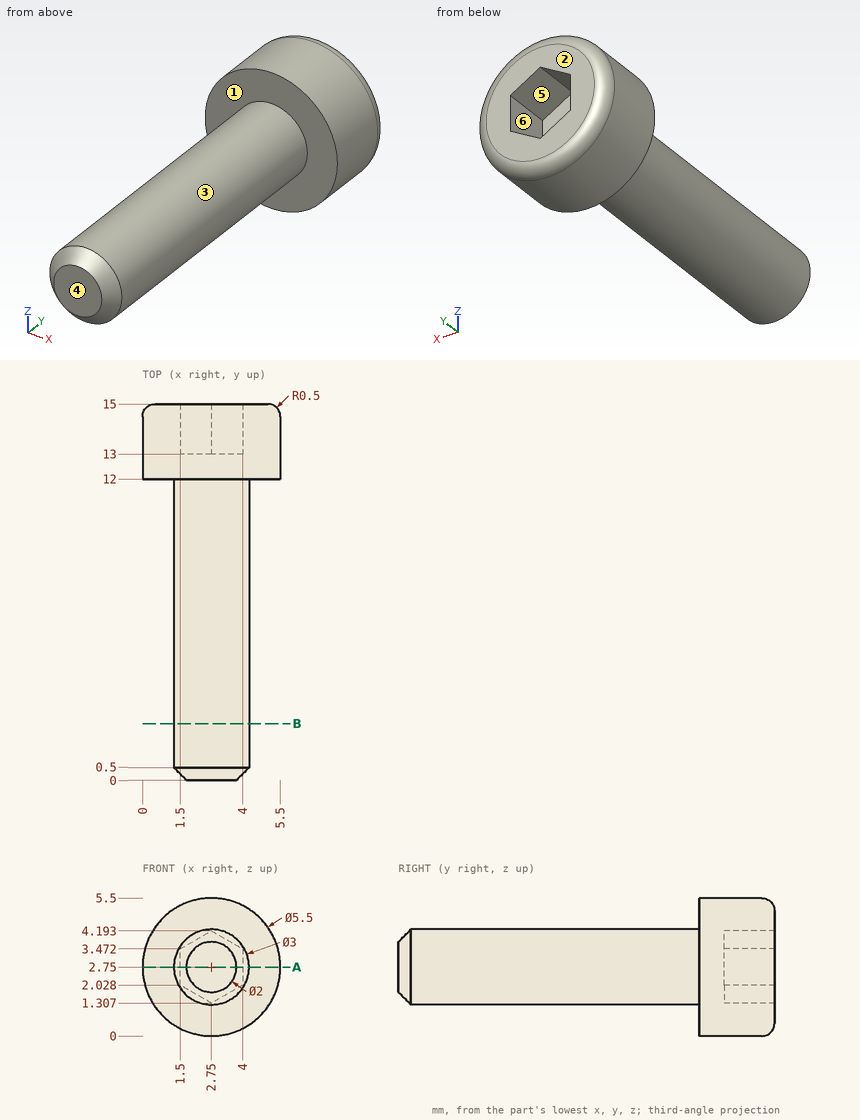
Can you work these out from the drawing? Everything is in mm from the part's minimum corner. A direction names the side the tool comes from. Round coordinates to 2 decimals unless told otherwise and drop trailing zeros. Loops run counter-clockwise (first coordinate to the right, second up) from the corner with the lowest first, then second, coordinate; pieces in that order, holes last. Notation, with made-up numbers: (-17.5, -19) - (19.5, -19) arc R20 ccw to (19.5, -3) - close; hole circle Ø7 at (35, -32). An arc over 180 degrees is marked (long way). One line per question, with ' | ' between items. Start each with the question number.
Q1. I want a section at B-B (y = 2.25). Write out the boundary of the cut face in (x, z).
Q2. Will these pins go through, and if not, where does the flat tip stop? pin 1 (0.8 mm diameter, centred on x = 2.5, z = 3.5, fed in from +Y); pin 2 (1.5 mm diameter, centred on x = 3, y = 2.5, fed in from +Z); pin 3 (1 mm diameter, centred on x = 1.5, y = 13.5, fed in from +Z).
Q3. Please list where these lines run through material, in increasing order: line 1 (Y direction, x = 3.8, z = 4); line 2 (X direction, y = 1.5, z = 2.8); line 3 (X direction, y = 14.5, z = 1.35) (1 decimal). Write a range as [from, to].
Q4. We'd pull the mould along Z, two halves only. Please class the marked faces 3, 4, 5 and 6: +Z half, -Z half, draft (parallel to the pull), parting line (faces both ways), or undercut.
Q5. I want a section at A-A (z = 2.75). Write out the boundary of the cut face in (x, y).
Q6. For the marked faces 1 and 2, which set-ups out of +Z, -Z, +X, -X, +Y, -Y let a thin tool reach every point of the face, with its end or its side?
Response values:
1) outline: circle Ø3 at (2.75, 2.75)
2) pin 1: stops at y = 13 | pin 2: stops at z = 4.25 | pin 3: stops at z = 5.4
3) line 1: y = [12, 15] | line 2: x = [1.25, 4.25] | line 3: x = [0.4, 2.7], [2.8, 5.1]
4) face 3: parting line | face 4: draft | face 5: undercut | face 6: undercut
5) outline: (0, 12) - (1.25, 12) - (1.25, 0.5) - (1.75, 0) - (3.75, 0) - (4.25, 0.5) - (4.25, 12) - (5.5, 12) - (5.5, 14.5) arc R0.5 ccw to (5, 15) - (4, 15) - (4, 13) - (1.5, 13) - (1.5, 15) - (0.5, 15) arc R0.5 ccw to (0, 14.5) - close
6) face 1: -Y | face 2: +Z, -Z, +X, -X, +Y
